Source: CAD feature listing. Evaluate the final solid. Frame: model axes, mm. Face numbers are marked on the shaded views. A direction names the side the tool comes from. Give positions to 0.01 mm unless a question says otherwise; leave off trailing zeros. Loops run counter-clockwise (first coordinate to the right, second up) from the corner with the lowest first, then second, coordinate; pieces in that order, holes last. Notation, with made-up numbers: (71, 61.5) -> (117, 61.5) arc R9 ccw to (117, 69.5) -> close; hole circle Ø1 at (2, -14.5). An arc over 180 degrees is marked (long way). Return JSON: item names as keys, results as strings. Group by question number.
(1) Pin query (flat end, axial travel): pin 1 (5 mm diameter, centred on x = 4.5, z = 3, fed in from -Y); pin 2 (5 mm diameter, centred on x = -0.5, z = 15.5, fed in from -Y); pin 3 (2.5 mm diameter, centred on x = 7.5, y = -30.5, fed in from -Z); pin 4 (3 mm diameter, centred on x = 5.5, y = -21, fed in from +Z). Return the tip coordinate at first contact, or that it passes through.
(2) Cut plane A-A on x = 0. Return loops of the section in (y, z).
(3) Cut plane C-C on y = 32. Return loops of the section in (x, z).
(4) Cut plane B-B on y = -2.5. Return loops of the section in (x, z), then the cut area to 3 significant figures.
(5) Access query for the marked faces 5, 6, 7, 8 and 9. Directions: +Z, -Z, +X, -X, +Y, -Y. A direction counts if a zero-diameter tool reaches every point of the face in a straight line with its end or side. Return the directions, or none.
(6) Ray query, line 1 (Z direction, x = 0, y = -13); line 2 (Y direction, x = -0.75, z = 17.25); line 3 (Y direction, x = 7, z = 16.5). Return the intervals inside material, ascending. Write a range as from..to.
(7) Draft query along X for the marked faces 1, 2, 3 and 4. Return one class per face: released by +X, released by -X, zero draft, split by the parting line, or undercut.
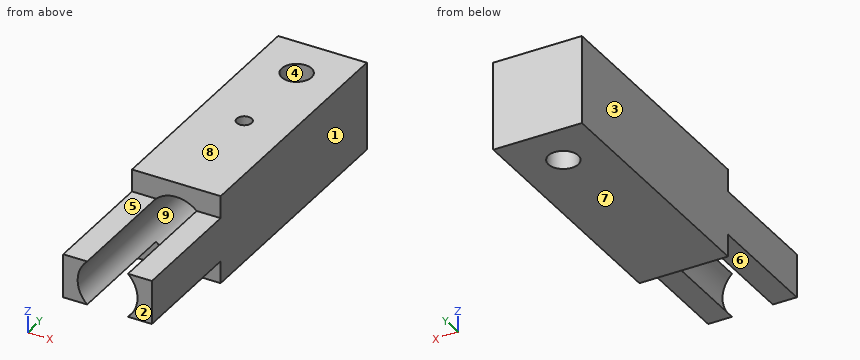
Autodesk Inventor part; units mm, degrees
ref_plane "YZ Plane" through (0, 0, 0) normal (1, 0, 0) x (0, 1, 0)
ref_plane "XZ Plane" through (0, 0, 0) normal (0, 1, 0) x (-1, 0, 0)
ref_plane "XY Plane" through (0, 0, 0) normal (0, 0, 1) x (1, 0, 0)
sketch "Sketch1" plane through (0, 0, 0) normal (0, 0, 1) x (1, 0, 0)
  line L0 (-9.398, -39.6875) -> (9.398, -39.6875)
  line L1 (9.398, -39.6875) -> (9.398, 39.6875)
  line L2 (9.398, 39.6875) -> (-9.398, 39.6875)
  line L3 (-9.398, 39.6875) -> (-9.398, -39.6875)
  line L4 (-9.398, -39.6875) -> (9.398, 39.6875) construction
  line L5 (9.398, -39.6875) -> (-9.398, 39.6875) construction
  point P0 (0, 0)
  dimension "d0" = 18.796
  dimension "d1" = 79.375
extrude "Extrusion1" add sketch "Sketch1" along normal blind 18.796
sketch "Sketch2" plane through (0, 0, 18.796) normal (0, 0, 1) x (1, 0, 0)
  circle A0 centre (0, 30.1625) radius 3.175
  line L0 (9.398, -39.6875) -> (9.398, 39.6875)
  line L1 (9.398, 39.6875) -> (-9.398, 39.6875)
  point P0 (0, 0)
  dimension "d4" = 6.35
  dimension "d5" = 9.398
  dimension "d6" = 9.525
extrude "Extrusion2" cut sketch "Sketch2" against normal blind 18.796
sketch "Sketch3" plane through (0, 0, 18.796) normal (0, 0, 1) x (1, 0, 0)
  circle A0 centre (0, 10.8077) radius 1.5875
  line L0 (9.398, -39.6875) -> (9.398, 39.6875)
  line L1 (9.398, 39.6875) -> (-9.398, 39.6875)
  point P0 (0, 0)
  dimension "d9" = 3.175
  dimension "d10" = 9.398
  dimension "d11" = 28.8798
extrude "Extrusion3" cut sketch "Sketch3" against normal blind 9.398
sketch "Sketch4" plane through (-9.398, -39.6875, 0) normal (0, -1, 0) x (1, 0, 0)
  circle A0 centre (9.398, 9.398) radius 6.35
  line L0 (18.796, 0) -> (18.796, 18.796)
  line L1 (0, 0) -> (18.796, 0)
  point P0 (9.398, 0)
  dimension "d14" = 12.7
  dimension "d15" = 9.398
  dimension "d16" = 9.398
extrude "Extrusion4" cut sketch "Sketch4" against normal blind 53.975
sketch "Sketch5" plane through (9.398, -39.6875, 0) normal (1, 0, 0) x (0, 0, -1)
  line L0 (-18.796, 79.375) -> (-18.796, 0)
  line L1 (-18.796, 0) -> (-14.0462, 0)
  line L2 (-14.0462, 0) -> (-14.0462, 25.4)
  line L3 (-14.0462, 25.4) -> (-18.796, 25.4)
  line L4 (-18.796, 25.4) -> (-18.796, 0)
  line L5 (0, 0) -> (-4.7498, 0)
  line L6 (-4.7498, 0) -> (-4.7498, 25.4)
  line L7 (-4.7498, 25.4) -> (0, 25.4)
  line L8 (0, 25.4) -> (0, 0)
  line L9 (0, 79.375) -> (-18.796, 79.375)
  line L10 (0, 0) -> (0, 79.375)
  point P0 (0, 39.6875)
  dimension "d19" = 53.975
  dimension "d20" = 4.7498
  dimension "d21" = 4.7498
  dimension "d22" = 0
extrude "Extrusion5" cut sketch "Sketch5" against normal blind 53.975
properties part number "Piston Block"
Answers:
{
 "1": {"pin 1": "y = -39.69", "pin 2": "y = -14.29", "pin 3": "z = 4.75", "pin 4": "z = 14.05"},
 "2": {"outline": "(-14.29, 0) -> (26.99, 0) -> (26.99, 18.8) -> (12.4, 18.8) -> (12.4, 15.75) -> (14.29, 15.75) -> (14.29, 3.05) -> (-14.29, 3.05) -> close; (-14.29, 15.75) -> (9.22, 15.75) -> (9.22, 18.8) -> (-14.29, 18.8) -> close; (33.34, 0) -> (39.69, 0) -> (39.69, 18.8) -> (33.34, 18.8) -> close"},
 "3": {"outline": "(-9.4, 0) -> (-2.59, 0) -> (-2.59, 18.8) -> (-9.4, 18.8) -> close; (2.59, 0) -> (9.4, 0) -> (9.4, 18.8) -> (2.59, 18.8) -> close"},
 "4": {"outline": "(-9.4, 0) -> (9.4, 0) -> (9.4, 18.8) -> (-9.4, 18.8) -> close; hole circle Ø12.7 at (0, 9.4)", "area": "227 mm²"},
 "5": {"face 5": "+Z, +X, -X, -Y", "face 6": "-Z, +X, -X, -Y", "face 7": "-Z, +X, -X, +Y, -Y", "face 8": "+Z, +X, -X, +Y, -Y", "face 9": "-Y"},
 "6": {"line 1": "0..3.05, 15.75..18.8", "line 2": "-14.29..9.41, 12.21..27.08, 33.25..39.69", "line 3": "-14.29..39.69"},
 "7": {"face 1": "released by +X", "face 2": "zero draft", "face 3": "released by -X", "face 4": "undercut"}
}
